Here's how the part is built. I have some questions about the finished solid (model axes, mm). Face numbers are marked on the shaded views. A direction names the side the tool comes from. Give positions to 0.01 mm unless a question says otherwise; leave off trailing zeros. Loops run counter-clockwise (first coordinate to the right, second up) from the corner with the lowest first, then second, coordinate; pieces in that order, holes last. Notation, with made-up numbers: (19.5, -19) - (42.5, -19) arc R22 ccw to (42.5, 12) - close; hole circle Ø11 at (-31.5, -11). An arc over 180 degrees is marked (long way). Put each result on its own line as item: value. Start each with the question number.
from build123d import *

# Parameters (mm, degrees)
SKETCH2_W           = 50
SKETCH2_H           = 35
BOSS_EXTRUDE1_DEPTH = 3.5
SKETCH3_R           = 1.85
CUT_EXTRUDE1_DEPTH  = 31.716445107
SKETCH5_R           = 3.5
BOSS_EXTRUDE2_DEPTH = 8


with BuildPart() as part:
    # Sketch2 → Boss-Extrude1 (new body)
    with BuildSketch(Plane(origin=(0, 0, 0), x_dir=(1, 0, 0), z_dir=(0, 1, 0))):
        Rectangle(SKETCH2_W, SKETCH2_H)
    extrude(amount=BOSS_EXTRUDE1_DEPTH)

    # Sketch3 → Cut-Extrude1 (cut, through all)
    with BuildSketch(Plane(origin=(0, 3.5, 0), x_dir=(1, 0, 0), z_dir=(0, 1, 0))):
        with Locations(Location((-16.6, 2.45, 0), (0, 0, 270))):
            Circle(SKETCH3_R)
        with Locations(Location((0, -8, 0), (0, 0, 270))):
            Circle(SKETCH3_R)
        with Locations(Location((16.6, 2.45, 0), (0, 0, 270))):
            Circle(SKETCH3_R)
    extrude(amount=-CUT_EXTRUDE1_DEPTH, mode=Mode.SUBTRACT)

    # Sketch5 → Boss-Extrude2 (add)
    with BuildSketch(Plane(origin=(8, 0, 0), x_dir=(0, 0, -1), z_dir=(1, 0, 0))):
        with BuildLine():
            Line((17.5, 3.5), (22.186446019, 4.416364401))
            ThreePointArc((22.186446019, 4.416364401), (27.235272499, -1.653328191), (19.401351351, -2.633887439))
            Line((19.401351351, -2.633887439), (17.5, 0))
            Line((17.5, 0), (17.5, 3.5))
        make_face()
        with Locations((23.05, 0)):
            Circle(SKETCH5_R, mode=Mode.SUBTRACT)
    boss_extrude2 = extrude(amount=BOSS_EXTRUDE2_DEPTH)

    # Mirror1: Boss-Extrude2 across plane
    add(boss_extrude2.mirror(Plane(origin=(0, 0, 0), x_dir=(0, 0, 1), z_dir=(1, 0, 0))))


solid = part.part
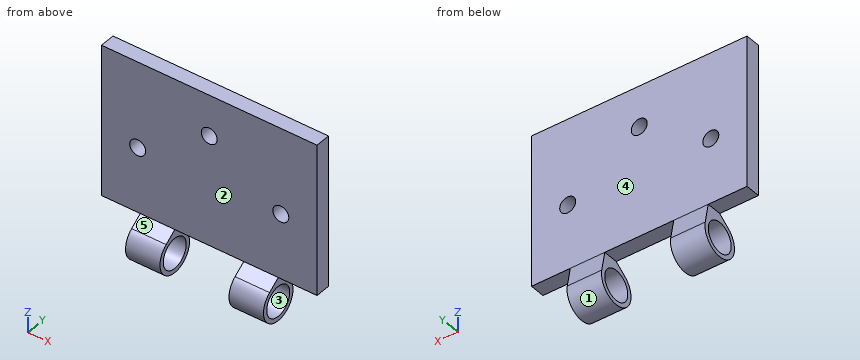
1) Which directions (+Z, -Z, +X, -X, +Y, -Y) give clear straight access to the entire face, cutting with the end or side of a thin tool? Please do the marked faces 1 and 2.
2) Suppose I cut it at D-D on z = 7.5. Please give me the cut outline in (x, y).
3) I need wall thicknesses on line 1 (X direction, y = 2.2, z = -2.45); line 2 (X direction, y = 2, z = -20); line 3 (Y direction, x = -14, z = -23.05). Which ranges of each line are inside material? Lowest first, please.
4) Thinking about a two-plate mould opening in Z: for the marked faces 3, 4 and 5, which applies, pulls with the +Z half, pulls with the -Z half, needs draft (parallel to the pull), parting line crosses it, or undercut?
5) Suppose I cut it at B-B on x = -16.6. Please give me the cut outline in (y, z), plus the area to 3 significant figures.
6) Suppose I cut it at A-A on y = 1.75. Please give me the cut outline in (x, z), plus the area to 3 significant figures.
7) I'm going to push flat-ended pins straight in: P1, Ø1, axis at x = -4, y = 2.5, coming from the -Z side; P2, Ø2.5, axis at y = 0, z = -20, coming from the +X side; P3, Ø4.5, axis at x = 16.6, z = -2.45, coming from the -Y side. Where does each tip first touch, or does it pass through?
8) Suppose I cut it at C-C on x = 14. Please give me the cut outline in (y, z), plus the area to 3 significant figures.
Ans:
1. face 1: +X, -X
1. face 2: +Z, +X, -X, -Y
2. outline: (-25, 0) - (-1.78, 0) - (-1.78, 3.5) - (-25, 3.5) - close; (1.78, 0) - (25, 0) - (25, 3.5) - (1.78, 3.5) - close
3. line 1: x = -25 to -18.45, -14.75 to 14.75, 18.45 to 25
3. line 2: x = -16 to -8, 8 to 16
3. line 3: y = -4.5 to -3.5, 3.5 to 4.5
4. face 3: undercut
4. face 4: needs draft
4. face 5: pulls with the +Z half
5. outline: (0, -17.5) - (3.5, -17.5) - (3.5, -4.3) - (0, -4.3) - close; (0, -0.6) - (3.5, -0.6) - (3.5, 17.5) - (0, 17.5) - close
5. area: 110 mm²
6. outline: (-25, -17.5) - (-16, -17.5) - (-16, -20.02) - (-8, -20.02) - (-8, -17.5) - (8, -17.5) - (8, -20.02) - (16, -20.02) - (16, -17.5) - (25, -17.5) - (25, 17.5) - (-25, 17.5) - close; (-16, -27.2) - (-8, -27.2) - (-8, -26.08) - (-16, -26.08) - close; (8, -27.2) - (16, -27.2) - (16, -26.08) - (8, -26.08) - close; hole circle Ø3.7 at (-16.6, -2.45); hole circle Ø3.7 at (0, 8); hole circle Ø3.7 at (16.6, -2.45)
6. area: 1,780 mm²
7. P1: stops at z = -17.5
7. P2: stops at x = 16
7. P3: stops at y = 0
8. outline: (-2.63, -19.4) arc R4.5 ccw (long way) to (4.42, -22.19) - (3.5, -17.5) - (3.5, 17.5) - (0, 17.5) - (0, -17.5) - close; hole circle Ø7 at (0, -23.05)
8. area: 155 mm²
